The listing builds one solid part. Answer for the finished solid, in the listing's coordinates (mm). A direction names the side the tool comes from. Give positions to 0.01 mm unless a question says otherwise; leave off trailing zeros. Write each question's results on one line, items separated by ' | '. Start each with the question number.
from build123d import *

# Parameters (mm, degrees)
F0_R     = 8.509
F1_DEPTH = 1.524
F2_R     = 4.191
F3_DEPTH = 3.556
F4_R     = 0.635
F5_SIZE  = 0.635


with BuildPart() as f1:
    # F0 (on Top) → F1 (new body)
    with BuildSketch(Plane.XY):
        Circle(F0_R)
    extrude(amount=F1_DEPTH)

    # F2 (on face) → F3 (join)
    with BuildSketch(Plane.XY.offset(1.524)):
        Circle(F2_R)
    extrude(amount=F3_DEPTH)

    # F4
    f4_edges = [f1.edges().sort_by_distance(p)[0] for p in [
        (-8.509, 0, 1.524),
        (8.509, 0, 0.762),
        (-8.509, 0, 0),
    ]]
    fillet(f4_edges, radius=F4_R)

    # F5
    f5_edges = [f1.edges().sort_by_distance(p)[0] for p in [
        (-4.191, 0, 5.08),
    ]]
    chamfer(f5_edges, length=F5_SIZE)

    # F6 (on Right) → F7 (revolve, cut)
    with BuildSketch(Plane.YZ):
        with BuildLine():
            Line((0, 0), (0, 1.905))
            ThreePointArc((0, 1.905), (-2.933456, 1.510415), (-5.658379, 0.354708))
            ThreePointArc((-5.658379, 0.354708), (-6.281844, 0.090282), (-6.953022, 0))
            Line((-6.953022, 0), (0, 0))
        make_face()
    revolve(axis=Axis((0, 0, 0.9525), (0, 0, 1)), mode=Mode.SUBTRACT)


solid = f1.part
1. Each of these flat-tipped pins is pushed along its axis until it touches: pin 1 Ø1 at (x, y) = (-2, 5.5) entering from +Z; pin 2 Ø8 at (x, y) = (3, -2.5) entering from +Z; pin 3 Ø1 at (x, z) = (-4.5, 1.5) entering from +Y; pin 4 Ø3 at (x, z) = (-6, 2.5) entering from +Y. Where does it stop, or does it pass through?
2. A tool of negligible diameter and unlimited length cuts with its end or side. For faces 1 (the flat face through (0, 0, 5.08)), 2 (the flat face through (3.4, -3.4, 1.524)), from which of +Z, -Z, +X, -X, +Y, -Y can it reach the whole face along a straight path? Write none if from no direction.
3. Consider probe 1 along Y at (x, z) = (-1.25, 0.45); probe 2 along Z at (x, y) = (-6.75, 3); probe 3 along Y at (x, z) = (-0.5, 0.6). Determine where each line is inside the solid, lowest interval first. Write a range as [from, to].
Results:
1) pin 1: stops at z = 1.52 | pin 2: stops at z = 5.08 | pin 3: stops at y = 7.37 | pin 4: stops at y = 6.62
2) face 1: +Z, +X, -X, +Y, -Y | face 2: +Z
3) probe 1: y = [-8.39, -5.35], [5.35, 8.39] | probe 2: z = [0, 1.52] | probe 3: y = [-8.49, -5.2], [5.2, 8.49]
